Here's how the part is built. I have some questions about the finished solid (model axes, mm). Coordinates: 2 decimals unless noted, no trailing zeros. Write each loop counter-clockwise with the first axis right and the second up, starting at its lowest first coordinate (ties: lowest second). Pieces come first, ordered by that corner, then holes.
Item 1: I want a section at A-A (x = 183.5). Please give me the cut outline in (y, z), and give its area (3 significant figures).
Item 2: I want a section at B-B (z = -65). Please give me the cut outline in (x, y).
Item 3: I'm going to push flat-ended pins straight in: P1, Ø1, axis at x = 278, y = 127.5, coming from the +Z side; P2, Ø0.6, axis at y = 128.5, z = -4.5, coming from the +X side; P3, Ø0.9, axis at x = 192.5, y = 127.5, coming from the -Z side. Where does each tip first touch, or does it pass through?
Item 4: I want a section at D-D (x = 227.5). Please give me the cut outline in (y, z).
Item 5: I want a section at C-C (y = 128.2). Count the separate pieces of the cut face and the enclosed holes in it, and give its area (3 significant figures).
Item 6: Please list where these lines run through material, in increasing order: line 1 (Z direction, x = 166, y = 127.4); line 2 (Z direction, x = 122.1, y = 128.3); line 3 (X direction, y = 128.6, z = -41).
from build123d import *

# Parameters (mm, degrees)
SKETCH_R   = 1.627
SKETCH_R_2 = 1.5
PAD_DEPTH  = 1.8542


with BuildPart() as part:
    # Sketch (on Face85 of Binder) → Pad (new body)
    with BuildSketch(Plane(origin=(0, 127.2271, 0), x_dir=(-1, 0, 0), z_dir=(0, 1, 0))):
        with BuildLine():
            Line((-330.3246, -11.1254), (-330.3246, -101.3746))
            ThreePointArc((-330.3246, -101.3746), (-329.973128, -102.223128), (-329.1246, -102.5746))
            Line((-329.1246, -102.5746), (-325.1852, -102.5746))
            ThreePointArc((-323.9852, -103.7746), (-324.336672, -102.926072), (-325.1852, -102.5746))
            Line((-323.9852, -110.4919), (-323.9852, -103.7746))
            ThreePointArc((-323.9852, -110.4919), (-320.25, -114.2271), (-316.5148, -110.4919))
            Line((-316.5148, -110.4919), (-316.5148, -103.7746))
            ThreePointArc((-315.3148, -102.5746), (-316.163328, -102.926072), (-316.5148, -103.7746))
            Line((-315.3148, -102.5746), (-111.6852, -102.5746))
            ThreePointArc((-110.4852, -103.7746), (-110.836672, -102.926072), (-111.6852, -102.5746))
            Line((-110.4852, -110.4919), (-110.4852, -103.7746))
            ThreePointArc((-110.4852, -110.4919), (-106.75, -114.2271), (-103.0148, -110.4919))
            Line((-103.0148, -110.4919), (-103.0148, -103.7746))
            ThreePointArc((-101.8148, -102.5746), (-102.663328, -102.926072), (-103.0148, -103.7746))
            Line((-101.8148, -102.5746), (-97.8754, -102.5746))
            ThreePointArc((-97.8754, -102.5746), (-97.026872, -102.223128), (-96.6754, -101.3746))
            Line((-96.6754, -101.3746), (-96.6754, -11.1254))
            ThreePointArc((-96.6754, -11.1254), (-97.026872, -10.276872), (-97.8754, -9.9254))
            Line((-97.8754, -9.9254), (-101.8148, -9.9254))
            ThreePointArc((-103.0148, -8.7254), (-102.663328, -9.573928), (-101.8148, -9.9254))
            Line((-103.0148, -2.0081), (-103.0148, -8.7254))
            ThreePointArc((-103.0148, -2.0081), (-106.75, 1.7271), (-110.4852, -2.0081))
            Line((-110.4852, -2.0081), (-110.4852, -8.7254))
            ThreePointArc((-111.6852, -9.9254), (-110.836672, -9.573928), (-110.4852, -8.7254))
            Line((-111.6852, -9.9254), (-315.3148, -9.9254))
            ThreePointArc((-316.5148, -8.7254), (-316.163328, -9.573928), (-315.3148, -9.9254))
            Line((-316.5148, -2.0081), (-316.5148, -8.7254))
            ThreePointArc((-316.5148, -2.0081), (-320.25, 1.7271), (-323.9852, -2.0081))
            Line((-323.9852, -2.0081), (-323.9852, -8.7254))
            ThreePointArc((-325.1852, -9.9254), (-324.336672, -9.573928), (-323.9852, -8.7254))
            Line((-325.1852, -9.9254), (-329.1246, -9.9254))
            ThreePointArc((-329.1246, -9.9254), (-329.973128, -10.276872), (-330.3246, -11.1254))
        make_face()
        with Locations((-320.25, -2.0081)):
            Circle(SKETCH_R, mode=Mode.SUBTRACT)
        with Locations((-106.75, -2.0081)):
            Circle(SKETCH_R, mode=Mode.SUBTRACT)
        with Locations((-122.1, -36.55)):
            Circle(SKETCH_R_2, mode=Mode.SUBTRACT)
        with Locations((-122.1, -75.95)):
            Circle(SKETCH_R_2, mode=Mode.SUBTRACT)
        with Locations((-106.75, -110.4919)):
            Circle(SKETCH_R, mode=Mode.SUBTRACT)
        with Locations((-320.25, -110.4919)):
            Circle(SKETCH_R, mode=Mode.SUBTRACT)
        with Locations((-274.5, -91.15)):
            Circle(SKETCH_R_2, mode=Mode.SUBTRACT)
        with Locations((-274.5, -21.35)):
            Circle(SKETCH_R_2, mode=Mode.SUBTRACT)
        with BuildLine():
            ThreePointArc((-326.1082, -24.579), (-327.1623, -23.5249), (-328.2164, -24.579))
            Line((-328.2164, -24.579), (-328.2164, -87.921))
            ThreePointArc((-328.2164, -87.921), (-327.1623, -88.9751), (-326.1082, -87.921))
            Line((-326.1082, -24.579), (-326.1082, -87.921))
        make_face(mode=Mode.SUBTRACT)
        with BuildLine():
            ThreePointArc((-98.7836, -24.579), (-99.8377, -23.5249), (-100.8918, -24.579))
            Line((-100.8918, -24.579), (-100.8918, -87.921))
            ThreePointArc((-100.8918, -87.921), (-99.8377, -88.9751), (-98.7836, -87.921))
            Line((-98.7836, -24.579), (-98.7836, -87.921))
        make_face(mode=Mode.SUBTRACT)
        with BuildLine():
            ThreePointArc((-303.6468, -12.0336), (-304.7009, -13.0877), (-303.6468, -14.1418))
            Line((-303.6468, -14.1418), (-240.3048, -14.1418))
            ThreePointArc((-240.3048, -14.1418), (-239.2507, -13.0877), (-240.3048, -12.0336))
            Line((-303.6468, -12.0336), (-240.3048, -12.0336))
        make_face(mode=Mode.SUBTRACT)
        with BuildLine():
            ThreePointArc((-186.6952, -12.0336), (-187.7493, -13.0877), (-186.6952, -14.1418))
            Line((-186.6952, -14.1418), (-123.3532, -14.1418))
            ThreePointArc((-123.3532, -14.1418), (-122.2991, -13.0877), (-123.3532, -12.0336))
            Line((-186.6952, -12.0336), (-123.3532, -12.0336))
        make_face(mode=Mode.SUBTRACT)
        with BuildLine():
            ThreePointArc((-303.6468, -98.3582), (-304.7009, -99.4123), (-303.6468, -100.4664))
            Line((-303.6468, -100.4664), (-240.3048, -100.4664))
            ThreePointArc((-240.3048, -100.4664), (-239.2507, -99.4123), (-240.3048, -98.3582))
            Line((-303.6468, -98.3582), (-240.3048, -98.3582))
        make_face(mode=Mode.SUBTRACT)
        with BuildLine():
            ThreePointArc((-186.6952, -98.3582), (-187.7493, -99.4123), (-186.6952, -100.4664))
            Line((-186.6952, -100.4664), (-123.3532, -100.4664))
            ThreePointArc((-123.3532, -100.4664), (-122.2991, -99.4123), (-123.3532, -98.3582))
            Line((-186.6952, -98.3582), (-123.3532, -98.3582))
        make_face(mode=Mode.SUBTRACT)
    extrude(amount=PAD_DEPTH)


solid = part.part
Answer:
1. outline: (127.23, -102.57) - (129.08, -102.57) - (129.08, -100.47) - (127.23, -100.47) - close; (127.23, -98.36) - (129.08, -98.36) - (129.08, -14.14) - (127.23, -14.14) - close; (127.23, -12.03) - (129.08, -12.03) - (129.08, -9.93) - (127.23, -9.93) - close
1. area: 164 mm2
2. outline: (96.68, 127.23) - (98.78, 127.23) - (98.78, 129.08) - (96.68, 129.08) - close; (100.89, 127.23) - (326.11, 127.23) - (326.11, 129.08) - (100.89, 129.08) - close; (328.22, 127.23) - (330.32, 127.23) - (330.32, 129.08) - (328.22, 129.08) - close
3. P1: stops at z = -9.93
3. P2: stops at x = 323.99
3. P3: stops at z = -102.57
4. outline: (127.23, -102.57) - (129.08, -102.57) - (129.08, -9.93) - (127.23, -9.93) - close
5. separate pieces: 1
5. enclosed holes: 14
5. area: 21,100 mm2
6. line 1: z = -102.57 to -100.47, -98.36 to -14.14, -12.03 to -9.93
6. line 2: z = -102.57 to -77.45, -74.45 to -38.05, -35.05 to -9.93
6. line 3: x = 96.68 to 98.78, 100.89 to 326.11, 328.22 to 330.32
